```python
from build123d import *

# Parameters (mm, degrees)
BOSS_EXTRUDE1_DEPTH      = 20
BOSS_EXTRUDE2_DEPTH      = 3
BOSS_EXTRUDE2_DEPTH_BACK = 3
SKETCH2_W                = 18
SKETCH2_H                = 21
SKETCH2_W_2              = 12
SKETCH2_H_2              = 15
BOSS_EXTRUDE3_DEPTH      = 21
CUT_EXTRUDE1_DEPTH       = 30
CUT_EXTRUDE1_DEPTH_BACK  = 30
SKETCH4_W                = 3
SKETCH4_H                = 1
FILLET1_R                = 1


with BuildPart() as part:
    # Sketch1 → Boss-Extrude1 (new body)
    with BuildSketch(Plane(origin=(0, 0, 0), x_dir=(1, 0, 0), z_dir=(0, 1, 0))):
        with BuildLine():
            Line((31.500049634, -86.559686407), (-9.212862555, -16.042853971))
            ThreePointArc((-9.212862555, -16.042853971), (-13.066315501, -13.096617855), (-16.02146997, -9.25))
            Line((-16.02146997, -9.25), (33.97853003, -95.852540378))
            ThreePointArc((33.97853003, -95.852540378), (32.124838484, -91.369992609), (31.500049634, -86.559686407))
        make_face()
        with BuildLine():
            Line((36.143593539, -94.602540378), (31.500049634, -86.559686407))
            ThreePointArc((31.500049634, -86.559686407), (32.124838484, -91.369992609), (33.97853003, -95.852540378))
            ThreePointArc((33.97853003, -95.852540378), (50, -105.102540378), (66.02146997, -95.852540378))
            ThreePointArc((66.02146997, -95.852540378), (67.869627786, -91.390692713), (68.5, -86.602540378))
            ThreePointArc((68.5, -86.602540378), (68.499987591, -86.581113379), (68.499950366, -86.559686407))
            Line((68.499950366, -86.559686407), (63.856406461, -94.602540378))
            ThreePointArc((63.856406461, -94.602540378), (50, -102.602540378), (36.143593539, -94.602540378))
        make_face()
        with BuildLine():
            ThreePointArc((116.02146997, -9.25), (113.066315501, -13.096617855), (109.212862555, -16.042853971))
            Line((109.212862555, -16.042853971), (68.499950366, -86.559686407))
            ThreePointArc((68.499950366, -86.559686407), (68.499987591, -86.581113379), (68.5, -86.602540378))
            ThreePointArc((68.5, -86.602540378), (67.869627786, -91.390692713), (66.02146997, -95.852540378))
            Line((66.02146997, -95.852540378), (116.02146997, -9.25))
        make_face()
        with BuildLine():
            ThreePointArc((100, 18.5), (95.191153985, 17.864070085), (90.712912189, 16))
            Line((90.712912189, 16), (100, 16))
            ThreePointArc((100, 16), (111.313708499, 11.313708499), (116, 0))
            ThreePointArc((116, 0), (115.454813221, -4.141104722), (113.856406461, -8))
            Line((113.856406461, -8), (109.212862555, -16.042853971))
            ThreePointArc((109.212862555, -16.042853971), (113.066315501, -13.096617855), (116.02146997, -9.25))
            ThreePointArc((116.02146997, -9.25), (117.869627786, -4.788152334), (118.5, 0))
            ThreePointArc((118.5, 0), (113.081475452, 13.081475452), (100, 18.5))
        make_face()
        with BuildLine():
            ThreePointArc((0, 18.5), (4.808846015, 17.864070085), (9.287087811, 16))
            Line((9.287087811, 16), (90.712912189, 16))
            ThreePointArc((90.712912189, 16), (95.191153985, 17.864070085), (100, 18.5))
            Line((100, 18.5), (0, 18.5))
        make_face()
        with BuildLine():
            ThreePointArc((-13.856406461, -8), (-13.856406461, 8), (0, 16))
            Line((0, 16), (9.287087811, 16))
            ThreePointArc((9.287087811, 16), (4.808846015, 17.864070085), (0, 18.5))
            ThreePointArc((0, 18.5), (-16.02146997, 9.25), (-16.02146997, -9.25))
            ThreePointArc((-16.02146997, -9.25), (-13.066315501, -13.096617855), (-9.212862555, -16.042853971))
            Line((-9.212862555, -16.042853971), (-13.856406461, -8))
        make_face()
    extrude(amount=BOSS_EXTRUDE1_DEPTH)



with BuildPart() as body_2:
    # Sketch2 → Boss-Extrude2 (new, two sides: drawn at the far end of the back side and taken through both)
    with BuildSketch(Plane.ZY.offset(-50).offset(-BOSS_EXTRUDE2_DEPTH_BACK)):
        with Locations((114.102540378, 10.5)):
            Rectangle(SKETCH2_W, SKETCH2_H)
        with Locations((114.102540378, 10.5)):
            Rectangle(SKETCH2_W_2, SKETCH2_H_2, mode=Mode.SUBTRACT)
    extrude(amount=BOSS_EXTRUDE2_DEPTH + BOSS_EXTRUDE2_DEPTH_BACK)


with BuildPart() as part_1:
    add(part.part)

    add(body_2.part)  # Boss-Extrude3 merges body 2
    # Sketch3 → Boss-Extrude3 (add)
    with BuildSketch(Plane(origin=(0, 21, 0), x_dir=(1, 0, 0), z_dir=(0, 1, 0))):
        Polygon((43, -103.727084168), (47, -106.727084168), (47, -105.102540378), (53, -105.102540378), (53, -106.727084168), (57, -103.727084168), align=None)
    extrude(amount=-BOSS_EXTRUDE3_DEPTH)

    # Sketch4 → Cut-Extrude1 (cut, two sides: drawn at the far end of the back side and taken through both)
    with BuildSketch(Plane.ZY.offset(-50).offset(-CUT_EXTRUDE1_DEPTH_BACK)):
        with Locations((105.227084168, 20.5)):
            Rectangle(SKETCH4_W, SKETCH4_H)
    extrude(amount=CUT_EXTRUDE1_DEPTH + CUT_EXTRUDE1_DEPTH_BACK, mode=Mode.SUBTRACT)

    # Fillet1
    fillet1_edges = [part_1.edges().sort_by_distance(p)[0] for p in [
        (50, 20, 106.727084168),
    ]]
    fillet(fillet1_edges, radius=FILLET1_R - 0.0001)  # a hair under: the kernel refuses the full size


solid = part_1.part
```
Verification items for the finished model (mm, model axes). A direction names the side the tool comes from. Give positions to 0.01 mm unless a question says otherwise; leave off trailing zeros. Order: outer loops, then holes, each group sorted by start corner. A loop starts at its lowest first (then second) coordinate and runs counter-clockwise, first axis right, second up. Notation, with made-up numbers: (68.25, 56.5) -> (86.25, 56.5) arc R27 cw to (86.25, 73.5) -> close; hole circle Ø5 at (87.25, -21.75). An arc over 180 degrees is marked (long way). One line per item, written item: value.
(1) Draft check along X on faces 1 (the face through (50.2, 9.9, 102.6)), 2 (the face through (49, 10, -16)), 3 (the face through (90.67, 9.86, 53.16)), 4 (the face through (50, 10, 123.103)). Enter one of: pulls with the +X half, pulls with the -X half, needs draft (parallel to the pull), parting line crosses it, or undercut.
Final values:
face 1: undercut
face 2: undercut
face 3: pulls with the +X half
face 4: needs draft
(2) Sectioned sample at C-C on x = 51. Count the separate pieces of the cut face and the enclosed holes in it, then the cut area to 3 significant figures.
Final values:
separate pieces: 2
enclosed holes: 1
area: 297 mm^2
(3) Tool access check on faces 5 (the face through (53, 10.6, 120.3)), 6 (the face through (47, 10.6, 120.3)), 7 (the face through (50, 18, 114)). Record the directions out of +Z, -Z, +X, -X, +Y, -Y that give a thin tool (end or side, any length) a straight path to the whole face; none if there is none.
Final values:
face 5: +Z, +X, +Y, -Y
face 6: +Z, -X, +Y, -Y
face 7: +X, -X
(4) Sectioned sample at A-A on y = 13.5. Record the cut outline in (x, z).
Final values:
outline: (-16.02, 9.25) arc R18.5 ccw to (0, -18.5) -> (100, -18.5) arc R18.5 ccw to (116.02, 9.25) -> (66.02, 95.85) arc R18.5 ccw to (57, 103.73) -> (53, 106.73) -> (53, 108.1) -> (47, 108.1) -> (47, 106.73) -> (43, 103.73) arc R18.5 ccw to (33.98, 95.85) -> close; (47, 120.1) -> (53, 120.1) -> (53, 123.1) -> (47, 123.1) -> close; hole (-13.86, 8) arc R16 ccw to (0, -16) -> (100, -16) arc R16 ccw to (113.86, 8) -> (63.86, 94.6) arc R16 ccw to (36.14, 94.6) -> close
(5) Scan lines: line 1 along X through (y, z) = (10, 68); line 2 along Z through (x, y) = (1, 19); line 3 along Z through (x, y) = (92, 9.5). Record each from-to range of solid material in increasing order. Write a range as [from, to].
Final values:
line 1: [17.9, 20.78], [79.22, 82.1]
line 2: [-18.5, -16], [33.73, 38.73]
line 3: [-18.5, -16], [45.86, 50.86]
(6) Sectioned sample at D-D on x = 86. Record the cut outline in (y, z), then the cut area to 3 significant figures.
Final values:
outline: (0, -18.5) -> (20, -18.5) -> (20, -16) -> (0, -16) -> close; (0, 56.25) -> (20, 56.25) -> (20, 61.25) -> (0, 61.25) -> close
area: 150 mm^2
(7) Sectioned sample at B-B on z = 110. Record the cut outline in (x, y), then the cut area to 3 significant figures.
Final values:
outline: (47, 0) -> (53, 0) -> (53, 3) -> (47, 3) -> close; (47, 18) -> (53, 18) -> (53, 21) -> (47, 21) -> close
area: 36.0 mm^2
(8) Gauge pin test, flat ends, axial feed: pin 1 (5 mm diameter, centred on y = 9.5, z = 74, fed in from -X); pin 2 (1 mm diameter, centred on x = 43.5, y = 3, fed in from +Z); pin 3 (4 mm diameter, centred on y = 7, z = 80.5, fed in from -X); pin 4 (1.5 mm diameter, centred on x = 12, z = 47.5, fed in from -Y). Record the tip position at first contact, or that the pin passes through.
Final values:
pin 1: x = 19.92
pin 2: z = 104.48
pin 3: x = 23.96
pin 4: through
